Answer from the drawing. Dimensions are ordinates in mm from the lowest x, y and z of the part. A direction names the side the tool comes from. Give positions to 0.01 mm unless a question says otherwise; leave off trailing zeros. Loops run counter-clockwise (first coordinate to the right, second up) from the corner with the lowest first, then second, coordinate; pieces in that order, holes last. Notation, with made-up numbers: (-24.75, 73.25) -> (14.25, 73.25) arc R5 cw to (14.25, 80.25) -> close; hole circle Ø4 at (64, 84). An arc over 180 degrees is marked (long way). Answer as CSV lines item,"result". Start each with the question number.
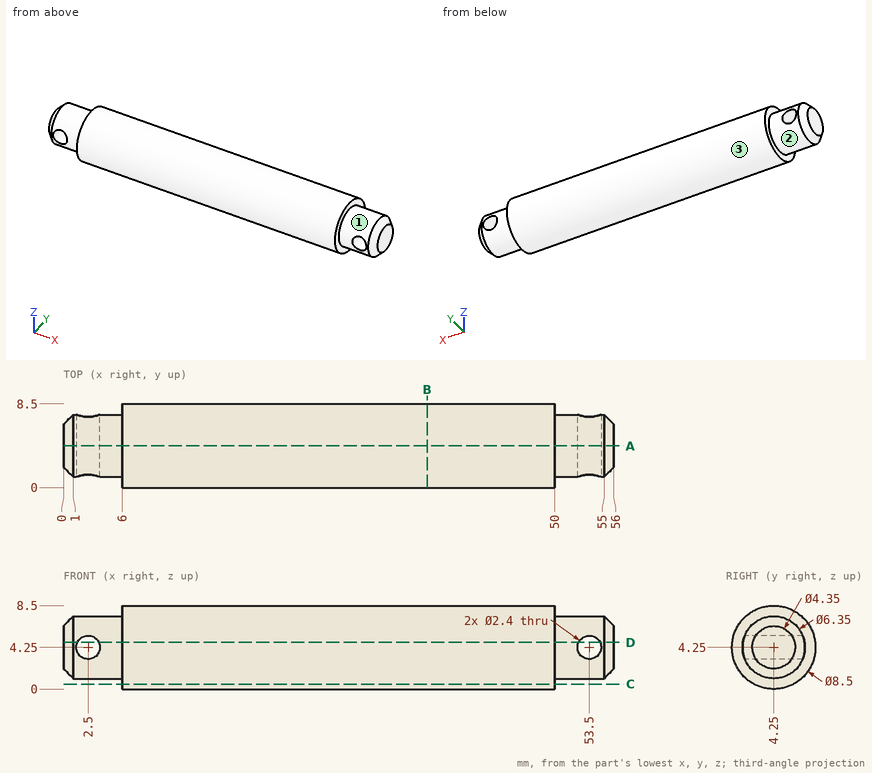
(1) Find section B-B on x = 37. Write down the section's boundary in (y, z), then the cut area to 3 significant figures.
(2) Find the intervals of material crossed by line 1 along X through (y, z) = (6.25, 4.25); line 2 along X through (y, z) = (6.25, 3.5); line 3 along Z through (x, y) = (53.5, 3), in increasing order. Write a range as from..to.
(3) Find section D-D on z = 4.75. Give the number of separate pieces and of enclosed holes in the cut face, then the cut area to 3 significant figures.
(4) Each of these flat-tipped pins is pushed along its axis until it touches: P1, Ø3, axis at x = 2.5, z = 4.25, coming from the +Y side (3 decimals); P2, Ø1.4, axis at x = 53.5, z = 4.25, coming from the -Y side; P3, Ø1, axis at y = 6.5, z = 1, coming from the -X side; P4, Ø1, axis at x = 18, z = 1.5, coming from the +Y side. Where does it stop, or does it pass through?
(5) Find section C-C on z = 0.5. Write down the section's boundary in (x, y), then the cut area to 3 significant figures.
(6) Find section A-A on y = 4.25. Write down the section's boundary in (x, z) (3 decimals).
(7) A tool of negligible diameter and unlimited length cuts with its end or side. For the marked faces 1, 2 and 3, from which of +Z, -Z, +X, -X, +Y, -Y can it reach the whole face along a straight path? Write none if from no direction.
Answer block:
1,outline,"circle Ø8.5 at (4.25, 4.25)"
1,area,"56.7 mm2"
2,line 1,"x = 0..1.3, 3.7..52.3, 54.7..56"
2,line 2,"x = 0..1.56, 3.44..52.56, 54.44..56"
2,line 3,"z = 1.33..3.05, 5.45..7.17"
3,separate pieces,"3"
3,enclosed holes,"0"
3,area,"417 mm2"
4,P1,"stops at y = 7.425"
4,P2,"passes through"
4,P3,"stops at x = 6"
4,P4,"stops at y = 7.86"
5,outline,"(6, 2.25) -> (50, 2.25) -> (50, 6.25) -> (6, 6.25) -> close"
5,area,"176 mm2"
6,outline,"(0, 2.075) -> (1, 1.075) -> (6, 1.075) -> (6, 0) -> (50, 0) -> (50, 1.075) -> (55, 1.075) -> (56, 2.075) -> (56, 6.425) -> (55, 7.425) -> (50, 7.425) -> (50, 8.5) -> (6, 8.5) -> (6, 7.425) -> (1, 7.425) -> (0, 6.425) -> close; hole circle Ø2.4 at (2.5, 4.25); hole circle Ø2.4 at (53.5, 4.25)"
7,face 1,"+X"
7,face 2,"-X"
7,face 3,"+X, -X"
